```python
from build123d import *

# Parameters (mm, degrees)
SKETCH_2_W      = 9.723167254
SKETCH_2_H      = 12
EXTRUDE_1_DEPTH = 2
SKETCH_3_R      = 4
SKETCH_3_R_2    = 2.5
EXTRUDE_2_DEPTH = 4
SKETCH_4_R      = 2
EXTRUDE_3_DEPTH = 7.4
FILLET_1_R      = 0.4


with BuildPart() as part:
    # Эскиз2 → Бобышка-Вытянуть1 (new body)
    with BuildSketch(Plane.XY):
        Rectangle(SKETCH_2_W, SKETCH_2_H)
    extrude(amount=EXTRUDE_1_DEPTH)

    # Эскиз3 → Бобышка-Вытянуть2 (add)
    with BuildSketch(Plane.XY.offset(2)):
        with Locations((-0.238416373, 0.5)):
            Circle(SKETCH_3_R)
        with Locations((-0.238416373, 0.5)):
            Circle(SKETCH_3_R_2, mode=Mode.SUBTRACT)
    extrude(amount=EXTRUDE_2_DEPTH)

    # Эскиз4 → Бобышка-Вытянуть3 (add)
    with BuildSketch(Plane(origin=(0, 0, 0), x_dir=(-1, 0, 0), z_dir=(0, 0, -1))):
        with Locations(Location((-2.861583627, 0.7, 0), (0, 0, 180))):
            Circle(SKETCH_4_R)
    extrude(amount=EXTRUDE_3_DEPTH)

    # Скругление1
    fillet_1_edges = [part.edges().sort_by_distance(p)[0] for p in [
        (-4.238416373, 0.5, 6),
    ]]
    fillet(fillet_1_edges, radius=FILLET_1_R)


solid = part.part
```
CAD build for the part. Positions are in the model's coordinates, mm. A direction names the side the tool comes from. Round coordinates to 2 decimals unless told otherwise and drop trailing zeros. Write each loop counter-clockwise with the first axis right and the second up, starting at its lowest first coordinate (ties: lowest second). Pieces come first, ordered by that corner, then holes. Notation, with made-up numbers: (27, 48.25) -> (34, 48.25) arc R20 ccw to (34, 68.25) -> close; hole circle Ø10 at (50, -2). An arc over 180 degrees is marked (long way). Answer in a Markdown table with one row per item. Add a question column.
Item 1: Saw through at C-C, the plane x = 4. Write the cut outline in (y, z), then the cut area to 3 significant figures.
Item 2: Saw through at D-D, the plane z = -4.25. Write the cut outline in (x, y).
Item 3: Mould opens along Y. For faces 1 (the face through (-0.56, 2.98, 3.97)), 2 (the face through (-4.862, 0, 1)), 3 (the face through (0.864, 0.612, -3.648)), 4 (the face through (0, 1, 2)) say: pulls with the +Y half, pulls with the -Y half, needs draft (parallel to the pull), parting line crosses it, or undercut.
Item 4: Drill centre lines: line 1 (Y direction, x = 2.75, z = -0.25); line 2 (Z direction, x = -0.5, y = 5.5); line 3 (Z direction, x = 2, y = -0.25). Where is each one in solid material? Low to high. Write a range as from..to.
Item 5: Drop flat-ended pins along their axis: pin 1 Ø2 at (x, z) = (-1, 4.5) entering from -Y; pin 2 Ø1 at (x, y) = (3.5, -3) entering from -Z; pin 3 Ø4 at (y, z) = (1, -2.5) entering from -X. Give the stop position or say it passes through.
Item 6: Which spindle directions (+Z, -Z, +X, -X, +Y, -Y) get a long thin tool onto all of the face, cutting with end or side? Do faces 5 (the face through (-1.106, -3.405, 3.775)), 6 (the face through (4.862, 0, 1)). Say none if no direction does.
Item 7: Saw through at A-A, the plane z = 3. Write the cut outline in (x, y).
Findings below:
| question | item | result |
|---|---|---|
| 1 | outline | (-6, 0) -> (-0.94, 0) -> (-0.94, -7.4) -> (2.34, -7.4) -> (2.34, 0) -> (6, 0) -> (6, 2) -> (-6, 2) -> close |
| 1 | area | 48.3 mm^2 |
| 2 | outline | circle Ø4 at (2.86, 0.7) |
| 3 | face 1 | undercut |
| 3 | face 2 | needs draft |
| 3 | face 3 | parting line crosses it |
| 3 | face 4 | undercut |
| 4 | line 1 | y = -1.3..2.7 |
| 4 | line 2 | z = 0..2 |
| 4 | line 3 | z = -7.4..2 |
| 5 | pin 1 | stops at y = -3.5 |
| 5 | pin 2 | stops at z = 0 |
| 5 | pin 3 | stops at x = 0.86 |
| 6 | face 5 | +Z |
| 6 | face 6 | +Z, -Z, +X, +Y, -Y |
| 7 | outline | circle Ø8 at (-0.24, 0.5); hole circle Ø5 at (-0.24, 0.5) |
